```python
from build123d import *

# Parameters (mm, degrees)
CROQUIS1_R              = 12.5
SALIENTE_EXTRUIR1_DEPTH = 24
CROQUIS2_W              = 7.746059902
CROQUIS2_H              = 14.16230267
CORTAR_EXTRUIR1_DEPTH   = 6
CROQUIS3_W              = 7.04155471
CROQUIS3_H              = 14.887858528
SALIENTE_EXTRUIR2_DEPTH = 5
CHAFL_N1_SIZE           = 1
CHAFL_N2_SIZE           = 1
CROQUIS4_R              = 1.75
CORTAR_EXTRUIR2_DEPTH   = 34.963215395
CHAFL_N3_SIZE           = 1
CROQUIS5_W              = 5.029681936
CROQUIS5_H              = 10.86411298
CORTAR_EXTRUIR3_DEPTH   = 30.008619409


with BuildPart() as part:
    # Croquis1 → Saliente-Extruir1 (new body)
    with BuildSketch(Plane.XY):
        Circle(CROQUIS1_R)
    extrude(amount=SALIENTE_EXTRUIR1_DEPTH)

    # Croquis2 → Cortar-Extruir1 (cut)
    with BuildSketch(Plane.XY.offset(24)):
        Rectangle(CROQUIS2_W, CROQUIS2_H)
    extrude(amount=-CORTAR_EXTRUIR1_DEPTH, mode=Mode.SUBTRACT)

    # Croquis3 → Saliente-Extruir2 (add)
    with BuildSketch(Plane(origin=(0, 0, 0), x_dir=(-1, 0, 0), z_dir=(0, 0, -1))):
        Rectangle(CROQUIS3_W, CROQUIS3_H)
    extrude(amount=SALIENTE_EXTRUIR2_DEPTH)

    # Chaflán1
    chafl_n1_edges = [part.edges().sort_by_distance(p)[0] for p in [
        (-3.520777355, 0, -5),
        (0, 7.443929264, -5),
        (3.520777355, 0, -5),
        (0, -7.443929264, -5),
    ]]
    chamfer(chafl_n1_edges, length=CHAFL_N1_SIZE)

    # Chaflán2
    chafl_n2_edges = [part.edges().sort_by_distance(p)[0] for p in [
        (-12.5, 0, 0),
    ]]
    chamfer(chafl_n2_edges, length=CHAFL_N2_SIZE)

    # Croquis4 → Cortar-Extruir2 (cut, through all)
    with BuildSketch(Plane.XY.offset(24)):
        with Locations((-7.875, 0)):
            Circle(CROQUIS4_R)
        with Locations((7.875, 0)):
            Circle(CROQUIS4_R)
    extrude(amount=-CORTAR_EXTRUIR2_DEPTH, mode=Mode.SUBTRACT)

    # Chaflán3
    chafl_n3_edges = [part.edges().sort_by_distance(p)[0] for p in [
        (-12.5, 0, 24),
    ]]
    chamfer(chafl_n3_edges, length=CHAFL_N3_SIZE)

    # Croquis5 → Cortar-Extruir3 (cut, through all)
    with BuildSketch(Plane.XY.offset(18)):
        Rectangle(CROQUIS5_W, CROQUIS5_H)
    extrude(amount=-CORTAR_EXTRUIR3_DEPTH, mode=Mode.SUBTRACT)


solid = part.part
```
Input: part model. Units: mm. Frame: model coordinates. A direction names the side the tool comes from. Round coordinates to 2 decimals unless told otherwise and drop trailing zeros. Order: outer loops, then holes, each group sorted by start corner. A loop starts at its lowest first (then second) coordinate and runs counter-clockwise, first axis right, second up. Notation, with made-up numbers: (-2, 64) - (29, 64) arc R35 ccw to (29, 101) - close; hole circle Ø9 at (81.25, 34). An arc over 180 degrees is marked (long way). One line per question, with ' | ' between items. Start each with the question number.
1) Ray query, probe 1 along Y at (x, z) = (-1, -2.25); probe 2 along Z at (x, y) = (0.5, 7.5); probe 3 along X at (y, z) = (-5.25, -1). Return the intervals inside material, ascending.
2) Cut plane D-D, the plane z = 17. Return the cut outline in (x, y) (3 decimals), then the cut area to 3 significant figures.
3) Pull-direction query (X, two-part tool) for faces 1 (the flat face through (3.873, 0, 21)), 2 (the cylindrical face through (11.923, 3.755, 11.846)), 3 (the flat face through (0, -6, -5)); classes: +X half, -X half, draft (parallel to the pull), parting line (faces both ways), or undercut.
4) Cut plane A-A, the plane x = 0. Return the cut outline in (y, z), then the cut area to 3 significant figures.
5) Cut plane B-B, the plane z = 20. Return the cut outline in (x, y) (3 decimals), then the cut area to 3 significant figures.
6) Set-up query: faces 4 (the flat face through (-3.873, 0, 21)), 5 (the flat face through (0, -7.444, -2)), 6 (the flat face through (0, -5.432, 7)). Return all of +Z, -Z, +X, -X, +Y, -Y with unobstructed straight access to the full face (end or side cutting, diameter ignored); none if empty.
7) Cut plane C-C, the plane y = 0. Give the number of separate pieces and of enclosed holes in the cut face, then the cut area to 3 significant figures.
8) Contact query for flat-ended pins moving along their axis: P1, Ø1.5, axis at x = 4, y = 8.5, coming from the -Z side; P2, Ø1.5, axis at x = -9, z = 6.5, coming from the -Y side; P3, Ø3.5, axis at y = 2, z = 11, coming from the +X side; P4, Ø3, axis at x = -7.875, y = 0, coming from the -Z side. Output: stop coordinate, or through.
Worked out:
1) probe 1: y = -7.44 to -5.43, 5.43 to 7.44 | probe 2: z = 0 to 24 | probe 3: x = -3.52 to -2.51, 2.51 to 3.52
2) outline: circle Ø25 at (0, 0); hole circle Ø3.5 at (-7.875, 0); hole (-2.515, -5.432) - (2.515, -5.432) - (2.515, 5.432) - (-2.515, 5.432) - close; hole circle Ø3.5 at (7.875, 0) | area: 417 mm^2
3) face 1: undercut | face 2: parting line | face 3: draft
4) outline: (-12.5, 1) - (-11.5, 0) - (-7.44, 0) - (-7.44, -4) - (-6.44, -5) - (-5.43, -5) - (-5.43, 18) - (-7.08, 18) - (-7.08, 24) - (-11.5, 24) - (-12.5, 23) - close; (5.43, -5) - (6.44, -5) - (7.44, -4) - (7.44, 0) - (11.5, 0) - (12.5, 1) - (12.5, 23) - (11.5, 24) - (7.08, 24) - (7.08, 18) - (5.43, 18) - close | area: 337 mm^2
5) outline: circle Ø25 at (0, 0); hole circle Ø3.5 at (-7.875, 0); hole (-3.873, -7.081) - (3.873, -7.081) - (3.873, 7.081) - (-3.873, 7.081) - close; hole circle Ø3.5 at (7.875, 0) | area: 362 mm^2
6) face 4: +Z | face 5: -Z, +X, -X, -Y | face 6: +Z, -Z
7) separate pieces: 4 | enclosed holes: 0 | area: 302 mm^2
8) P1: stops at z = 0 | P2: stops at y = -9.39 | P3: stops at x = 12.5 | P4: passes through
